Could you check a few things on this drawing? It's one solid part, dimensions in mm from its lowest x, y, z. A direction names the side the tool comes from. Round coordinates to 2 decimals unless told otherwise and drop trailing zeros. Order: outer loops, then holes, each group sorted by start corner. A loop starts at its lowest first (then second) coordinate and runs counter-clockwise, first axis right, second up. Notation, with made-up numbers: M 57,39 L 90,39 A16 cw 90,48 Z; hole C 38.25,49.5 d1. An arc over 180 degrees is marked long. Answer as CSV lines item,"result". Start each with the question number.
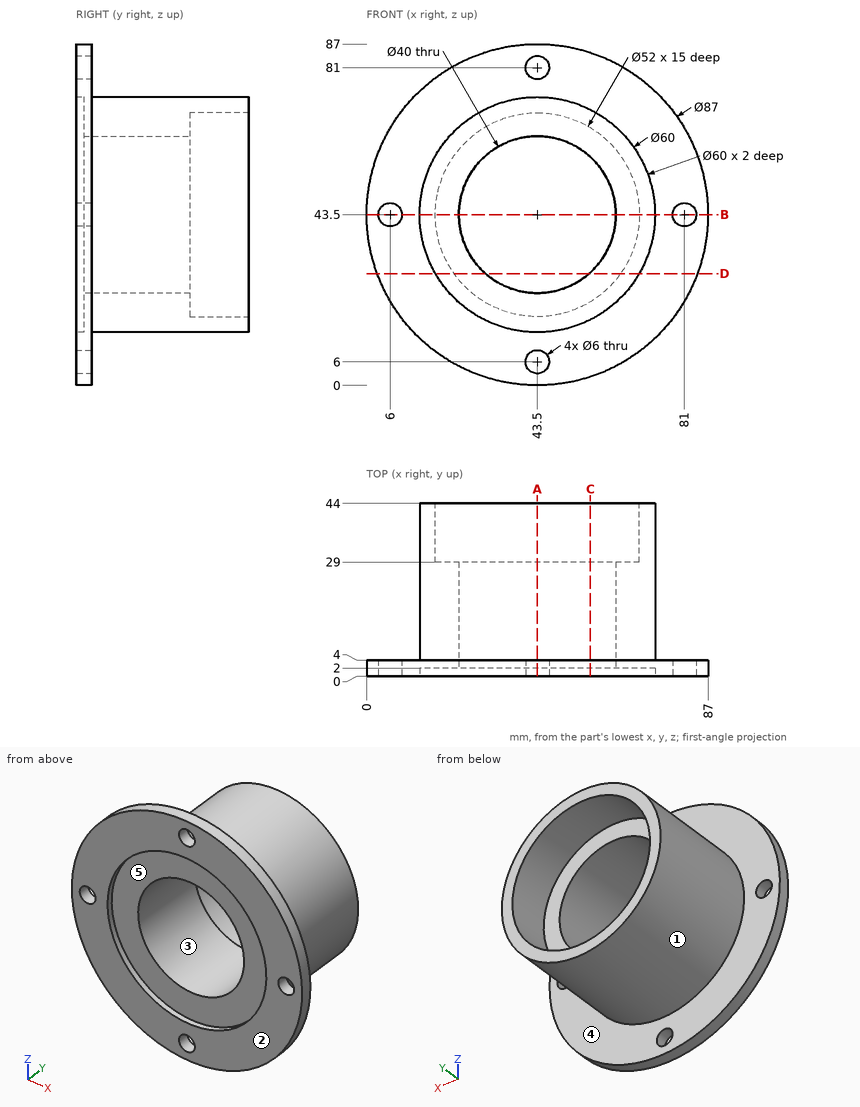
Item 1: If I drill on line 1 along X through (y, z) = (1, 43.5); line 2 along X through (y, z) = (37, 42.5); line 3 along Y through (x, z) = (57, 6), over which ranges is the centre line in solid material (lowest first)?
Item 2: If we section it at C-C on x = 57: Please give me the cut outline in (y, z), and give its area (3 significant figures).
Item 3: We'd pull the mould along Z, two halves only. Please class the marked faces 1, 2 and 3: pulls with the +Z half, pulls with the -Z half, needs draft (parallel to the pull), parting line crosses it, or undercut.
Item 4: If we section it at A-A on x = 43.5: Please give me the cut outline in (y, z), and give its area (3 significant figures).
Item 5: For P1, Ø3.5, axis at x = 81, z = 43.5, coming from the -Y side; P2, Ø4, axis at x = 21.5, y = 7, coming from the -Z side; P3, Ø1.5, axis at y = 8, z = 57, coming from the +X side; P4, Ø2, axis at y = 20, z = 70.5, coming from the +X side, each with a flat end and sliding along its axis, tell me the tip position at first contact or that it passes through.
Item 6: If we section it at D-D on z = 28.5: Please give me the cut outline in (x, y), and give its area (3 significant figures).
Item 7: If we section it at B-B on z = 43.5: Please give me the cut outline in (x, y).
Item 8: Which directions (+Z, -Z, +X, -X, +Y, -Y) give clear straight access to the entire face, cutting with the end or side of a thin tool? Please do the marked faces 4 and 5.
Geometry says:
1,line 1,"0 to 3, 9 to 13.5, 73.5 to 78, 84 to 87"
1,line 2,"13.52 to 17.52, 69.48 to 73.48"
1,line 3,"0 to 4"
2,outline,"M 0,2.15 L 4,2.15 L 4,16.71 L 44,16.71 L 44,21.28 L 29,21.28 L 29,28.74 L 2,28.74 L 2,16.71 L 0,16.71 Z; M 0,70.29 L 2,70.29 L 2,58.26 L 29,58.26 L 29,65.72 L 44,65.72 L 44,70.29 L 4,70.29 L 4,84.85 L 0,84.85 Z"
2,area,"903 mm²"
3,face 1,"parting line crosses it"
3,face 2,"needs draft"
3,face 3,"undercut"
4,outline,"M 0,0 L 4,0 L 4,3 L 0,3 Z; M 0,9 L 4,9 L 4,13.5 L 44,13.5 L 44,17.5 L 29,17.5 L 29,23.5 L 2,23.5 L 2,13.5 L 0,13.5 Z; M 0,73.5 L 2,73.5 L 2,63.5 L 29,63.5 L 29,69.5 L 44,69.5 L 44,73.5 L 4,73.5 L 4,78 L 0,78 Z; M 0,84 L 4,84 L 4,87 L 0,87 Z"
4,area,"720 mm²"
5,P1,"through"
5,P2,"z = 21.14"
5,P3,"x = 70.66"
5,P4,"x = 58.47"
6,outline,"M 2.67,0 L 17.52,0 L 17.52,2 L 30.27,2 L 30.27,29 L 22.26,29 L 22.26,44 L 17.52,44 L 17.52,4 L 2.67,4 Z; M 56.73,2 L 69.48,2 L 69.48,0 L 84.33,0 L 84.33,4 L 69.48,4 L 69.48,44 L 64.74,44 L 64.74,29 L 56.73,29 Z"
6,area,"950 mm²"
7,outline,"M 0,0 L 3,0 L 3,4 L 0,4 Z; M 9,0 L 13.5,0 L 13.5,2 L 23.5,2 L 23.5,29 L 17.5,29 L 17.5,44 L 13.5,44 L 13.5,4 L 9,4 Z; M 63.5,2 L 73.5,2 L 73.5,0 L 78,0 L 78,4 L 73.5,4 L 73.5,44 L 69.5,44 L 69.5,29 L 63.5,29 Z; M 84,0 L 87,0 L 87,4 L 84,4 Z"
8,face 4,"+Y"
8,face 5,"-Y"
